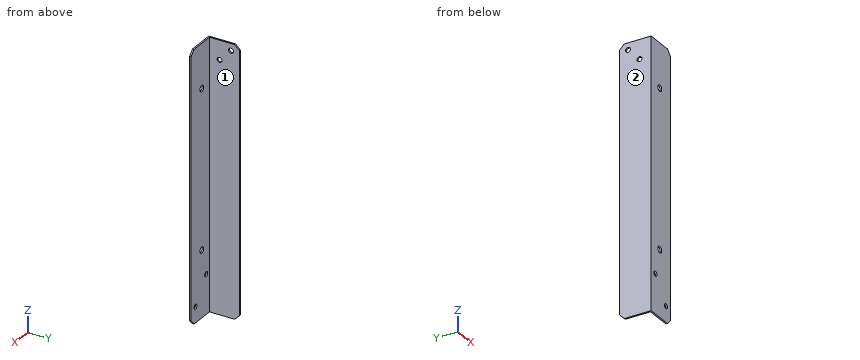
from build123d import *

# Parameters (mm, degrees)
BASE_DEPTH           = 170
CHAMFER1_SIZE        = 3
SKETCH4_R            = 1.55
CARRIAGESIDE_DEPTH   = 173.002906952
SKETCH6_R            = 1.55
CABLECHAINSIDE_DEPTH = 1
SKETCH7_R            = 2
CUT_EXTRUDE1_DEPTH   = 173.336879396


with BuildPart() as part:
    # Sketch1 → Base (new body)
    with BuildSketch(Plane.XY):
        Polygon((0, 0), (20, 0), (20, 1), (1, 1), (1, 20), (0, 20), align=None)
    extrude(amount=BASE_DEPTH)

    # Chamfer1
    chamfer1_edges = [part.edges().sort_by_distance(p)[0] for p in [
        (20, 0.5, 170),
        (0.5, 20, 170),
        (0.5, 20, 0),
        (20, 0.5, 0),
    ]]
    chamfer(chamfer1_edges, length=CHAMFER1_SIZE)

    # Sketch4 → CarriageSide (cut, through all)
    with BuildSketch(Plane(origin=(2, 1, 0), x_dir=(0, 0, -1), z_dir=(0, 1, 0))):
        with Locations(Location((-10, -13.5, 0), (0, 0, 90))):
            Circle(SKETCH4_R)
        with Locations(Location((-25, -2.5, 0), (0, 0, 90))):
            Circle(SKETCH4_R)
    extrude(amount=-CARRIAGESIDE_DEPTH, mode=Mode.SUBTRACT)

    # Sketch6 → CableChainSide (cut)
    with BuildSketch(Plane(origin=(1, 0, 0), x_dir=(0, 0, -1), z_dir=(1, 0, 0))):
        with Locations(Location((-165.6, 14.68, 0), (0, 0, 90))):
            Circle(SKETCH6_R)
        with Locations(Location((-157.8, 7.38, 0), (0, 0, 90))):
            Circle(SKETCH6_R)
    extrude(amount=-CABLECHAINSIDE_DEPTH, mode=Mode.SUBTRACT)

    # Sketch7 → Cut-Extrude1 (cut, through all)
    with BuildSketch(Plane.XZ):
        with Locations(Location((9, 142, 0), (0, 0, 270))):
            Circle(SKETCH7_R)
        with Locations(Location((9, 42, 0), (0, 0, 270))):
            Circle(SKETCH7_R)
    extrude(amount=-CUT_EXTRUDE1_DEPTH, mode=Mode.SUBTRACT)


solid = part.part
Geometry: final body of the model. Coordinates: model frame, mm. Face numbers are marked on the shaded views. A direction names the side the tool comes from. Round coordinates to 2 decimals unless told otherwise and drop trailing zeros. Loops run counter-clockwise (first coordinate to the right, second up) from the corner with the lowest first, then second, coordinate; pieces in that order, holes last. Notation, with made-up numbers: (70.5, 14.25) -> (91.5, 14.25) arc R34 cw to (91.5, 48.25) -> close; hole circle Ø3 at (30.5, 4.5). An arc over 180 degrees is marked (long way). One line per question, with ' | ' between items. Start each with the question number.
1. Set-up query: the marked faces 1 and 2. Return all of +Z, -Z, +X, -X, +Y, -Y with unobstructed straight access to the full face (end or side cutting, diameter ignored); none if empty.
2. Line query: line 1 along X through (y, z) = (0.8, 42); line 2 along Z through (x, y) = (0.25, 7.38); line 3 along Y through (x, z) = (0.35, 165.6). Output: solid intervals per line, ascending. Write a range as [from, to].
3. Section B-B on x = 15.5. Output: boundary loops of the cut face in (y, z).
4. Section A-A on z = 157.8. Output: boundary loops of the cut face in (x, y).
5. Section C-C on y = 7.38. Output: boundary loops of the cut face in (x, z).
6. Section D-D on z = 21.5. Output: boundary loops of the cut face in (x, y).
7. Contact query for flat-ended pins moving along their axis: pin 1 (12 mm diameter, centred on y = 6.5, z = 17, fed in from -X); pin 2 (9.5 mm diameter, centred on y = 8, z = 76.5, fed in from +X); pin 3 (10 mm diameter, centred on x = 16, z = 74.5, fed in from +Y); pin 4 (8 mm diameter, centred on x = 5.5, y = 15, fed in from +Z). Output: stop coordinate, or through.
Returned:
1) face 1: +Z, -Z, +X, +Y | face 2: +Z, -Z, -X, +Y, -Y
2) line 1: x = [0, 7], [11, 20] | line 2: z = [0, 156.25], [159.35, 170] | line 3: y = [0, 13.13], [16.23, 20]
3) outline: (0, 0) -> (1, 0) -> (1, 8.45) -> (0, 8.45) -> close; (0, 11.55) -> (1, 11.55) -> (1, 170) -> (0, 170) -> close
4) outline: (0, 0) -> (20, 0) -> (20, 1) -> (1, 1) -> (1, 5.83) -> (0, 5.83) -> close; (0, 8.93) -> (1, 8.93) -> (1, 20) -> (0, 20) -> close
5) outline: (0, 0) -> (1, 0) -> (1, 156.25) -> (0, 156.25) -> close; (0, 159.35) -> (1, 159.35) -> (1, 170) -> (0, 170) -> close
6) outline: (0, 0) -> (20, 0) -> (20, 1) -> (1, 1) -> (1, 20) -> (0, 20) -> close
7) pin 1: stops at x = 0 | pin 2: stops at x = 1 | pin 3: stops at y = 1 | pin 4: passes through
